Geometry: final body of the model. Coordinates: model frame, mm. A direction names the side the tool comes from. Round coordinates to 2 decimals unless told otherwise and drop trailing zeros. Loops run counter-clockwise (first coordinate to the right, second up) from the corner with the lowest first, then second, coordinate; pieces in that order, holes last. Notation, with made-up numbers: (-23, 21.5) - (4, 21.5) arc R22 cw to (4, 41.5) - close; hole circle Ø10 at (42, 79). An arc over 180 degrees is marked (long way). Answer as CSV lines item,"result".
from build123d import *

# Parameters (mm, degrees)
F1_DEPTH = 5
F2_R     = 0.7543712854
F3_DEPTH = 5
F5_DEPTH = 1


# Not quite as in the source:
# - a feature names something its author has since deleted; it is built from what else it names


with BuildPart() as f1:
    # F0 (on Right) → F1 (new body)
    with BuildSketch(Plane.YZ):
        Polygon((-18.8395921141, 32.0152118802), (-23.9240508527, 44.5727854967), (-23.9400436678, 39.4980984787), (-22.0310017467, 32.8367650509), (-18.6073519289, 24.5797261596), (-15.8885698766, 17.3296425492), (-15.8885698766, 15.8192086965), (-19.4129161537, 10.4823429137), (-22.0608360687, 8.8354363138), (-22.1316963434, 5.0447816029), (-16.7948305607, 6.5552145243), (-12.4649200588, 9.0726036578), (-9.0412702411, 12.1941678226), (-7.0434443557, 15.421631052), (-5.4162289016, 20.4512067139), (-7.732226979, 17.128251493), (-6.221793592, 20.4512067139), (-5.1141423173, 23.8748565316), (-5.1141423173, 26.6943331808), (-6.0204025358, 31.5277203918), (-7.732226979, 33.8437184691), (-7.0273578167, 30.722156167), (-7.732226979, 25.3852903843), (-10.4510085657, 21.3574655354), (-9.0412702411, 25.0832028687), (-8.2357050851, 28.3054616302), (-9.0412702411, 33.8437184691), (-11.1558772624, 38.4757146239), (-16.1906573921, 42.4028448761), (-13.4509364143, 39.5833663642), (-12.666311115, 36.0590219498), (-13.4509364143, 33.4521867335), (-15.3669025749, 29.7400020063), (-17.0433744788, 27.2252950817), align=None)
        Polygon((-23.9400436678, 39.4980984787), (-23.9240508527, 44.5727854967), (-26.5623033047, 38.9791950583), (-30.8922119439, 27.3992009461), (-32.8054279089, 29.9165919423), (-35.0207313895, 33.8437184691), (-35.0207313895, 37.4687612057), (-34.114472568, 40.6910181046), (-32.4026457965, 42.8056269884), (-35.0207313895, 40.6910181046), (-37.9520406538, 37.2414154054), (-39.350643754, 33.1388488412), (-39.350643754, 27.4998974055), (-37.7395115793, 21.659553051), (-40.6596846879, 26.492940262), (-41.4149016142, 30.2186775953), (-40.6596846879, 33.7430238724), (-41.4652489126, 32.5346775353), (-42.1701185405, 29.9165919423), (-43.169213802, 25.8295247582), (-42.1701185405, 22.5658137351), (-40.6596846879, 17.6317300647), (-42.7742935717, 20.4512067139), (-40.5589900911, 14.0066882595), (-36.631859839, 9.5760822296), (-31.5034037335, 6.6433727204), (-26.5623033047, 5.0447816029), (-25.1525640488, 8.7705180049), (-27.9720406979, 9.8781688139), (-30.6908208877, 12.697645463), (-32.3019511998, 15.7185140997), (-32.3019511998, 17.3296425492), (-29.885256663, 23.572769016), (-26.6505166424, 31.5225556516), (-26.6505166424, 32.8367650509), align=None)
        Polygon((-22.1316963434, 5.0447816029), (-22.0608360687, 8.8354363138), (-23.1386516243, 9.2739956453), (-23.1386516243, 14.6031556651), (-25.0721577589, 14.0031509837), (-25.1525640488, 8.7705180049), (-26.5623033047, 5.0447816029), align=None)
        Polygon((-23.1386516243, 20.699724555), (-23.9442177117, 38.1736308336), (-24.6739685535, 31.1146955937), (-24.6739685535, 24.4254041463), (-24.6739685535, 18.4981841594), (-27.4682287127, 21.715817973), (-25.7342918677, 17.5339697332), (-30.516512692, 16.6353452951), (-25.8594118059, 15.5345760286), (-28.1243625509, 12.1047943952), (-25.0721577589, 14.0031509837), (-23.1386516243, 14.6031556651), (-20.6095892936, 12.0629183948), (-22.0608360687, 15.7039240003), (-17.9000031203, 16.6353452951), (-22.0608360687, 17.6514387131), (-21.0862746716, 21.6422008803), (-23.1386516243, 18.5343166173), align=None)
    extrude(amount=F1_DEPTH)

    # F2 (on face) → F3 (cut)
    with BuildSketch(Plane.YZ.offset(5)):
        with Locations((-23.9965710789, 41.7759902775)):
            Circle(F2_R)
    extrude(amount=-F3_DEPTH, mode=Mode.SUBTRACT)

    # F4 (on face) → F5 (cut)
    with BuildSketch(Plane.YZ.offset(5)):
        Polygon((-16.5610130304, 11.6452822793), (-16.0314254463, 9.2795155942), (-15.6742927399, 9.4880603932), (-15.9501638263, 10.7204280794), (-15.5902979895, 10.9956199303), (-14.5742027089, 10.3393923491), (-14.309595339, 10.5828316882), (-16.2962192383, 11.8211973459), align=None)
        Polygon((-15.7808158547, 11.1649697646), (-16.056008637, 10.9638674185), (-16.1724351346, 11.2602282315), (-16.0208165755, 11.319792172), align=None, mode=Mode.SUBTRACT)
        Polygon((-15.2138965204, 12.3287355527), (-14.0034528449, 10.9638674185), (-13.7453717467, 11.1927486014), (-14.5170884397, 12.0629183948), (-13.149023056, 11.563308537), (-12.8642125055, 11.759115383), (-13.6474408209, 13.3967734873), (-13.9450938452, 13.192137459), (-13.3804315701, 11.9905229658), (-14.9350901603, 12.5759970916), align=None)
        Polygon((-13.31801555, 13.93365104), (-13.4715074673, 13.610381633), (-12.7293292628, 13.2944049069), (-12.5892657792, 13.6233913674), align=None)
        Polygon((-12.5892657792, 13.6233913674), (-12.7293292628, 13.2944049069), (-12.3227360628, 13.1213009442), (-12.1738159695, 13.4465167705), align=None)
        Polygon((-12.3227360628, 13.1213009442), (-12.7293292628, 13.2944049069), (-13.0343568597, 12.5779444352), (-12.6627200979, 12.3788343877), align=None)
        Polygon((-12.1738159695, 13.4465167705), (-12.3227360628, 13.1213009442), (-11.6736432537, 12.8449546173), (-11.5335797702, 13.1739410778), align=None)
        Polygon((-12.3115735045, 14.2756455901), (-12.5892657792, 13.6233913674), (-12.1738159695, 13.4465167705), (-11.8785644276, 14.0912952688), align=None)
        Polygon((-11.4597871365, 15.568957784), (-12.3322671279, 14.8386247456), (-11.0684223473, 13.5925812647), (-10.2732402928, 14.3991234958), align=None)
        Polygon((-11.7448461242, 14.678419102), (-11.3710323349, 15.0522328913), (-10.8014121652, 14.4826127216), (-11.1752259545, 14.1087989323), align=None, mode=Mode.SUBTRACT)
    extrude(amount=-F5_DEPTH, mode=Mode.SUBTRACT)


solid = f1.part
(1) Pin query (flat end, axial travel): P1, Ø0.6, axis at x = 2.5, z = 20, coming from the +Y side; P2, Ø1.5, axis at x = 1.5, z = 13, coming from the +Y side; P3, Ø1.4, axis at x = 2, z = 32, coming from the +Y side. Return the tip coordinate at first contact, or that it passes through.
Findings below:
P1,"y = -5.47"
P2,"y = -8.08"
P3,"y = -5.98"
(2) Section B-B (x = 1.4). Give the number of separate pieces and of enclosed holes in the cut face, and give its area (3 significant figures).
Findings below:
separate pieces,"1"
enclosed holes,"2"
area,"708 mm2"
(3) Section A-A (z = 19). Output: boundary loops of the cut face in (x, y), and give its area (3 significant figures).
Findings below:
outline,"(0, -42.28) - (5, -42.28) - (5, -41.69) - (0, -41.69) - close; (0, -41.08) - (5, -41.08) - (5, -31.66) - (0, -31.66) - close; (0, -26.34) - (5, -26.34) - (5, -25.11) - (0, -25.11) - close; (0, -24.67) - (5, -24.67) - (5, -23.14) - (0, -23.14) - close; (0, -22.83) - (5, -22.83) - (5, -21.73) - (0, -21.73) - close; (0, -16.51) - (5, -16.51) - (5, -6.88) - (0, -6.88) - close; (0, -6.43) - (5, -6.43) - (5, -5.89) - (0, -5.89) - close"
area,"120 mm2"
(4) Material intervals for line 1 along Y through (x, z) = (0.85, 10.5); line 2 along Y through (x, z) = (1.1, 35); line 3 along Y through (x, z) = (1.95, 39), sorted ascending.
Findings below:
line 1,"-37.45 to -28.57, -25.13 to -23.14, -19.4 to -10.9"
line 2,"-38.72 to -35.02, -28.05 to -25.77, -24.27 to -23.8, -22.65 to -20.05, -12.99 to -9.57"
line 3,"-36.46 to -34.59, -26.55 to -24.14, -23.8 to -21.67, -13.32 to -11.83"
(5) Access query for faces 5 (the face through (2, -39.351, 30)), 6 (the face through (4, -12.5, 13.3)), 7 (the face through (2.465, -25.314, 36.121)), 8 (the face through (5, -11.3, 14.6)), 9 (the face through (2.46, -6.24, 17.9)). Directions: +Z, -Z, +X, -X, +Y, -Y. A direction counts if a zero-diameter tool reaches every point of the face in a straight line with its end or side. Return the directions, or none.
Findings below:
face 5,"+Z, +X, -X"
face 6,"+X"
face 7,"+X, -X"
face 8,"+Z, -Z, +X, +Y, -Y"
face 9,"-Z, +X, -X, +Y"
(6) Draft query along Z for faces 1 (the face through (2.465, -19.951, 17.136)), 2 (the face through (2.46, -5.56, 29.08)), 3 (the face through (2.46, -19.5, 5.79)), 4 (the face through (2.46, -9.07, 23.4)). Return one class per face: pulls with the +Z half, pulls with the -Z half, needs draft (parallel to the pull), parting line crosses it, or undercut.
Findings below:
face 1,"undercut"
face 2,"pulls with the +Z half"
face 3,"pulls with the -Z half"
face 4,"undercut"
